from build123d import *

# Parameters (mm, degrees)
SKETCH1_W               = 10
SKETCH1_H               = 100
CUT_EXTRUDE1_REACH      = 63.237
CUT_EXTRUDE1_END_RADIUS = 25
SKETCH2_W               = 10
SKETCH2_H               = 20
CIRPATTERN1_COUNT       = 6


with BuildPart() as part:
    # Sketch1 → Revolve1 (revolve)
    with BuildSketch(Plane.XY, mode=Mode.PRIVATE) as revolve1_sk:
        with Locations((-20, 0)):
            Rectangle(SKETCH1_W, SKETCH1_H)
    revolve(revolve1_sk.sketch.rotate(Axis((0, 56.451612903, 0), (0, -1, 0)), 270), axis=Axis((0, 56.451612903, 0), (0, -1, 0)))

    # Cut-Extrude1: up to this cylinder (the profile starts inside it)
    cut_extrude1_end = Plane(origin=(0, 0, 0), z_dir=(0, 1, 0)) * Cylinder(CUT_EXTRUDE1_END_RADIUS, 177.474, mode=Mode.PRIVATE)
    # Sketch2 → Cut-Extrude1 (cut, up to the surface)
    with BuildSketch(Plane.XY, mode=Mode.PRIVATE) as cut_extrude1_sk1:
        Rectangle(SKETCH2_W, SKETCH2_H)
    cut_extrude1_tool1 = extrude(cut_extrude1_sk1.sketch, amount=-CUT_EXTRUDE1_REACH, mode=Mode.PRIVATE) & cut_extrude1_end
    cut_extrude1 = cut_extrude1_tool1.solids().sort_by_distance((0, 0, 0))[0]
    add(cut_extrude1, mode=Mode.SUBTRACT)

    # CirPattern1: Cut-Extrude1 ×6 about axis
    cirpattern1_axis = Axis((0, 0, 0), (0, 1, 0))
    for i in range(1, CIRPATTERN1_COUNT):
        add(cut_extrude1.rotate(cirpattern1_axis, i * 360 / CIRPATTERN1_COUNT), mode=Mode.SUBTRACT)


solid = part.part
Source: CAD feature listing. Evaluate the final solid. Frame: model axes, mm. A direction names the side the tool comes from. Round coordinates to 2 decimals unless told otherwise and drop trailing zeros. Loops run counter-clockwise (first coordinate to the right, second up) from the corner with the lowest first, then second, coordinate; pieces in that order, holes last. Notation, with made-up numbers: (56.5, 3) -> (112.5, 3) arc R17 cw to (112.5, 22) -> close; hole circle Ø3 at (-27, -37). An arc over 180 degrees is marked (long way). Answer as a JSON object with one key per item and string values. Group by question number.
Q1. Section query C-C (z = 0). Output: boundary loops of the cut face in (x, y).
Q2. Access query for faces 1 (the flat face through (17, -10, 10)), 2 (the flat face through (14.168, -0.14, 13.953)), 3 (the cylindrical face through (5.745, 0.7, 13.856)), 4 (the flat face through (0, -10, 19)). Directions: +Z, -Z, +X, -X, +Y, -Y. A direction counts if a zero-diameter tool reaches every point of the face in a straight line with its end or side. Return the directions, or none.
Q3. Section query D-D (y = -31.5). Output: boundary loops of the cut face in (x, z), plus the area to 3 significant figures.
Q4. Section query A-A (x = 0). Output: boundary loops of the cut face in (y, z).
Q5. Ray query, line 1 (Z direction, x = 15.5, y = 8.5); line 2 (X direction, y = 29, z = 0); line 3 (Y direction, x = -18.5, z = 9). Return the intervals inside material, ascending. Write a range as from..to.
Q6. Contact query for flat-ended pins moving along their axis: P1, Ø3, axis at y = 1.5, z = 18, coming from the -X side; P2, Ø5, axis at y = -24, z = -4.5, coming from the -X side; P3, Ø10, axis at y = 22, z = -4.5, coming from the -X side. Output: stop coordinate, or through.
Q7. Mould query, pull axis Z, two halves, no side actions, for faces 5 (the flat face through (17, 10, -10)), 6 (the flat face through (14.168, -0.14, -13.953)), 7 (the flat face through (0, -10, -19)). Classes: pulls with the +Z half, pulls with the -Z half, needs draft (parallel to the pull), parting line crosses it, or undercut.
Q8. Section query B-B (y = -4). Output: boundary loops of the cut face in (x, z).
Completed:
{
 "1": {"outline": "(-25, -50) -> (-15, -50) -> (-15, 50) -> (-25, 50) -> close; (15, -50) -> (25, -50) -> (25, 50) -> (15, 50) -> close"},
 "2": {"face 1": "none", "face 2": "+X", "face 3": "+Y, -Y", "face 4": "+Z, -Z"},
 "3": {"outline": "circle Ø50 at (0, 0); hole circle Ø30 at (0, 0)", "area": "1,260 mm²"},
 "4": {"outline": "(-50, -25) -> (-10, -25) -> (-10, -15) -> (-50, -15) -> close; (-50, 15) -> (-10, 15) -> (-10, 25) -> (-50, 25) -> close; (10, -25) -> (50, -25) -> (50, -15) -> (10, -15) -> close; (10, 15) -> (50, 15) -> (50, 25) -> (10, 25) -> close"},
 "5": {"line 1": "-19.62..-14.72, -3.18..3.18, 14.72..19.62", "line 2": "-25..-15, 15..25", "line 3": "-50..-10, 10..50"},
 "6": {"P1": "x = -18.71", "P2": "x = -24.92", "P3": "x = -25"},
 "7": {"face 5": "undercut", "face 6": "undercut", "face 7": "needs draft"},
 "8": {"outline": "(-23.71, -7.92) -> (-14.75, -2.74) arc R15 cw to (-14.75, 2.74) -> (-23.71, 7.92) arc R25 ccw to start; (-18.71, -16.58) arc R25 ccw to (-5, -24.49) -> (-5, -14.14) arc R15 cw to (-9.75, -11.4) -> close; (-18.71, 16.58) -> (-9.75, 11.4) arc R15 cw to (-5, 14.14) -> (-5, 24.49) arc R25 ccw to start; (5, -24.49) arc R25 ccw to (18.71, -16.58) -> (9.75, -11.4) arc R15 cw to (5, -14.14) -> close; (5, 14.14) arc R15 cw to (9.75, 11.4) -> (18.71, 16.58) arc R25 ccw to (5, 24.49) -> close; (14.75, -2.74) -> (23.71, -7.92) arc R25 ccw to (23.71, 7.92) -> (14.75, 2.74) arc R15 cw to start"}
}
